```python
from build123d import *

# Parameters (mm, degrees)
SKETCH_25_R              = 10.043747569
EXTRUDE_13_DEPTH         = 280
SKETCH_26_R              = 16.505129475
CUT_EXTRUDE_3_DEPTH      = 336.875889274
CUT_EXTRUDE_4_DEPTH      = 336.875889274
CUT_EXTRUDE_4_DEPTH_BACK = 336.875889274
SKETCH_27_W              = 70.665536313
SKETCH_27_H              = 50
SKETCH_27_W_2            = 68.866777207


with BuildPart() as part:
    # 草图25 → 凸台-拉伸13 (new body)
    with BuildSketch(Plane.XY):
        with BuildLine():
            Line((0, -20.387033345), (183.674687946, -22.201454999))
            Line((183.674687946, -22.201454999), (183.674687946, -5.617235602))
            Line((183.674687946, -5.617235602), (19.597902766, -5.617235602))
            ThreePointArc((19.597902766, -5.617235602), (-12.27013364, 16.281122476), (0, -20.387033345))
        make_face()
        Circle(SKETCH_25_R, mode=Mode.SUBTRACT)
    extrude(amount=EXTRUDE_13_DEPTH)

    # 草图26 → 切除-拉伸3 (cut, through all)
    with BuildSketch(Plane(origin=(0, -5.617235602, 0), x_dir=(1, 0, 0), z_dir=(0, 1, 0))):
        with Locations(Location((88.997396182, -50, 0), (0, 0, 270))):
            Circle(SKETCH_26_R)
        with Locations(Location((96.350965064, -230, 0), (0, 0, 270))):
            Circle(SKETCH_26_R)
    extrude(amount=-CUT_EXTRUDE_3_DEPTH, mode=Mode.SUBTRACT)

    # 草图27 → 切除-拉伸4 (cut, two sides: drawn at the far end of the back side and taken through both)
    with BuildSketch(Plane(origin=(0, -5.617235602, 0), x_dir=(1, 0, 0), z_dir=(0, 1, 0)).offset(-CUT_EXTRUDE_4_DEPTH_BACK)):
        with Locations((-6.880817282, -55)):
            Rectangle(SKETCH_27_W, SKETCH_27_H)
        with Locations((-7.780196834, -155)):
            Rectangle(SKETCH_27_W_2, SKETCH_27_H)
        with Locations((-7.780196834, -255)):
            Rectangle(SKETCH_27_W_2, SKETCH_27_H)
    extrude(amount=CUT_EXTRUDE_4_DEPTH + CUT_EXTRUDE_4_DEPTH_BACK, mode=Mode.SUBTRACT)


solid = part.part
```
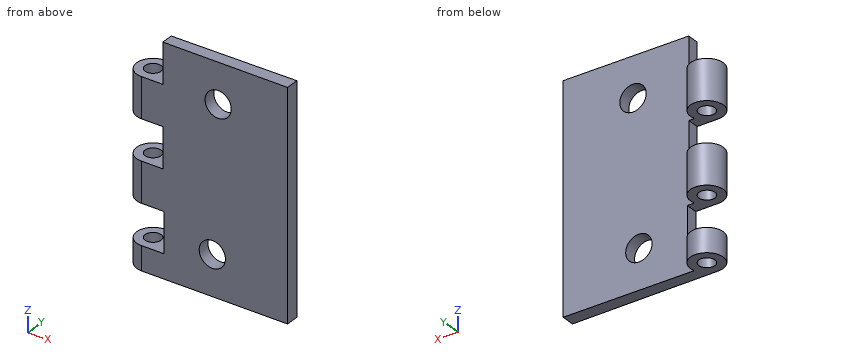
Part model, mm, in its own coordinate system. Round coordinates to 2 decimals unless told otherwise and drop trailing zeros. Order: outer loops, then holes, each group sorted by start corner. A loop starts at its lowest first (then second) coordinate and runs counter-clockwise, first axis right, second up. Notation, with made-up numbers: M -18,51.5 L 15,51.5 A17 cw 15,73.5 Z; hole C -3.75,82.5 d11. An arc over 180 degrees is marked long. Answer in a Markdown table with one row per item. Add a question column.
Q1. Cut at D-D on y = 14.5. Give the cut face in (x, z), and give its area (3 significant figures).
Q2. Cut at A-A on y = 0. Give the cut face in (x, z), and give its area (3 significant figures).
Q3. Cut at B-B on z = 96. Give the cut face in (x, y).
Q4. Pin check, flat tips, straight feed: pin 1 (16 mm diameter, centred on x = 0, y = 0, fed in from -Z); pin 2 (8 mm diameter, centred on y = -16.5, z = 145, fed in from -X); pin 3 (12.5 mm diameter, centred on x = 4, y = -5.5, fed in from +Z); pin 4 (12 mm diameter, centred on y = -14.5, z = 52, fed in from -X). Stop position of each tip, or through.
Q5. Wall check: L1, parallel to Z at x = 2, y = 16; L2, parallel to Y at x = 0, z = 195. Give the ranges that are in metal, low to high. Write a range as from..to.
Q6. Cut at C-C on z = 222. Give the cut face in (x, y).
Established:
| question | item | result |
|---|---|---|
| 1 | outline | M -14.33,0 L 14.33,0 L 14.33,30 L -14.33,30 Z; M -14.33,80 L 14.33,80 L 14.33,130 L -14.33,130 Z; M -14.33,180 L 14.33,180 L 14.33,230 L -14.33,230 Z |
| 1 | area | 3,730 mm2 |
| 2 | outline | M -20.39,0 L -10.04,0 L -10.04,30 L -20.39,30 Z; M -20.39,80 L -10.04,80 L -10.04,130 L -20.39,130 Z; M -20.39,180 L -10.04,180 L -10.04,230 L -20.39,230 Z; M 10.04,0 L 20.39,0 L 20.39,30 L 10.04,30 Z; M 10.04,80 L 20.39,80 L 20.39,130 L 10.04,130 Z; M 10.04,180 L 20.39,180 L 20.39,230 L 10.04,230 Z |
| 2 | area | 2,690 mm2 |
| 3 | outline | M 0,-20.39 L 183.67,-22.2 L 183.67,-5.62 L 19.6,-5.62 A20.39 ccw long Z; hole C 0,0 d20.09 |
| 4 | pin 1 | passes through |
| 4 | pin 2 | stops at x = 26.65 |
| 4 | pin 3 | stops at z = 230 |
| 4 | pin 4 | stops at x = 28.45 |
| 5 | L1 | z = 0..30, 80..130, 180..230 |
| 5 | L2 | y = -20.39..-10.04, 10.04..20.39 |
| 6 | outline | M 0,-20.39 L 81.91,-21.2 L 81.91,-5.62 L 19.6,-5.62 A20.39 ccw long Z; M 110.79,-21.48 L 183.67,-22.2 L 183.67,-5.62 L 110.79,-5.62 Z; hole C 0,0 d20.09 |
